from build123d import *

# Parameters (mm, degrees)
BOSS_EXTRUDE1_DEPTH = 12.7
SKETCH2_R           = 6.35
CUT_EXTRUDE5_DEPTH  = 12.7
FILLET1_R           = 2.54
FILLET2_R           = 2.54
SKETCH3_R           = 6.35
CUT_EXTRUDE6_DEPTH  = 12.7


with BuildPart() as part:
    # Sketch1 → Boss-Extrude1 (new body)
    with BuildSketch(Plane(origin=(0, 0, 0), x_dir=(1, 0, 0), z_dir=(0, 1, 0))):
        Polygon((0, 0), (203.2, 0), (101.6, 203.197957893), align=None)
    extrude(amount=BOSS_EXTRUDE1_DEPTH)

    # Sketch2 → Cut-Extrude5 (cut)
    with BuildSketch(Plane(origin=(0, 0, 0), x_dir=(1, 0, 0), z_dir=(0, 1, 0))):
        with Locations(Location((101.6, 165.097957893, 0), (0, 0, 270))):
            Circle(SKETCH2_R)
        Polygon((38.1, 25.4), (88.9, 25.4), (88.9, 127), align=None)
        Polygon((165.1, 25.4), (114.3, 25.4), (114.3, 127), align=None)
    extrude(amount=CUT_EXTRUDE5_DEPTH, mode=Mode.SUBTRACT)

    # Fillet1
    fillet1_edges = [part.edges().sort_by_distance(p)[0] for p in [
        (101.6, 6.35, -203.197957893),
        (203.2, 6.35, 0),
        (0, 6.35, 0),
    ]]
    fillet(fillet1_edges, radius=FILLET1_R)

    # Fillet2
    fillet2_edges = [part.edges().sort_by_distance(p)[0] for p in [
        (38.1, 6.35, -25.4),
        (88.9, 6.35, -25.4),
        (88.9, 6.35, -127),
        (165.1, 6.35, -25.4),
        (114.3, 6.35, -127),
        (114.3, 6.35, -25.4),
    ]]
    fillet(fillet2_edges, radius=FILLET2_R)

    # Sketch3 → Cut-Extrude6 (cut)
    with BuildSketch(Plane(origin=(0, 12.7, 0), x_dir=(1, 0, 0), z_dir=(0, 1, 0))):
        with Locations(Location((101.6, 88.9, 0), (0, 0, 270))):
            Circle(SKETCH3_R)
    extrude(amount=-CUT_EXTRUDE6_DEPTH, mode=Mode.SUBTRACT)


solid = part.part
Input: part model. Units: mm. Frame: model coordinates. A direction names the side the tool comes from. Give positions to 0.01 mm unless a question says otherwise; leave off trailing zeros. Order: outer loops, then holes, each group sorted by start corner. A loop starts at its lowest first (then second) coordinate and runs counter-clockwise, first axis right, second up. Notation, with made-up numbers: (-37, 28.5) -> (-15, 28.5) arc R35 cw to (-15, 65.5) -> close; hole circle Ø8 at (61, -14.75). An arc over 180 degrees is marked (long way). Use one line per item in the form item = value.
1) First-contact query: pin 1 Ø4 at (y, z) = (8, -60.5) entering from -X; pin 2 Ø1 at (y, z) = (10.5, -30) entering from -X; pin 3 Ø6 at (y, z) = (5.5, -165.5) entering from -X; pin 4 Ø11.5 at (x, z) = (101.6, -165.1) entering from +Y. Flat tips, straight axial feed; report the tip coordinate or a pass-through.
Response values:
pin_1 = 29.25
pin_2 = 14.75
pin_3 = 81.25
pin_4 = through
2) Mould query, pull axis X, two halves, no side actions, for faces 1 (the flat face through (100, 6, 0)), 2 (the flat face through (51.266, 6.261, -102.53)), 3 (the flat face through (153.3, 6.3, -99.8)), 4 (the flat face through (62.3, 6.3, -73.8)). Classes: pulls with the +X half, pulls with the -X half, needs draft (parallel to the pull), parting line crosses it, or undercut.
Response values:
face_1 = needs draft
face_2 = pulls with the -X half
face_3 = pulls with the +X half
face_4 = undercut
3) Section B-B, the plane y = 8. Return loops of the section in (x, z).
Response values:
outline = (1.84, -3.68) -> (99.33, -198.65) arc R2.54 ccw to (103.87, -198.65) -> (201.36, -3.68) arc R2.54 ccw to (199.09, 0) -> (4.11, 0) arc R2.54 ccw to start; hole (39.94, -29.08) -> (84.09, -117.38) arc R2.54 ccw to (88.9, -116.24) -> (88.9, -27.94) arc R2.54 ccw to (86.36, -25.4) -> (42.21, -25.4) arc R2.54 ccw to start; hole circle Ø12.7 at (101.6, -165.1); hole circle Ø12.7 at (101.6, -88.9); hole (114.3, -116.24) arc R2.54 ccw to (119.11, -117.38) -> (163.26, -29.08) arc R2.54 ccw to (160.99, -25.4) -> (116.84, -25.4) arc R2.54 ccw to (114.3, -27.94) -> close
4) Reachability of faces 5 (the flat face through (101, 0, -71)), 6 (the flat face through (140.9, 6.3, -73.8)) from +Z, -Z, +X, -X, +Y, -Y: full face, straight path, thin tool, end or side. Return the list, or none.
Response values:
face_5 = +Z, -Z, +X, -X, -Y
face_6 = +Y, -Y
5) Section C-C, the plane z = -47. Return loops of the section in (x, y).
Response values:
outline = (23.5, 0) -> (48.9, 0) -> (48.9, 12.7) -> (23.5, 12.7) -> close; (88.9, 0) -> (114.3, 0) -> (114.3, 12.7) -> (88.9, 12.7) -> close; (154.3, 0) -> (179.7, 0) -> (179.7, 12.7) -> (154.3, 12.7) -> close
6) Section D-D, the plane z = -88.9. Return loops of the section in (x, y).
Response values:
outline = (44.45, 0) -> (69.85, 0) -> (69.85, 12.7) -> (44.45, 12.7) -> close; (88.9, 0) -> (95.25, 0) -> (95.25, 12.7) -> (88.9, 12.7) -> close; (107.95, 0) -> (114.3, 0) -> (114.3, 12.7) -> (107.95, 12.7) -> close; (133.35, 0) -> (158.75, 0) -> (158.75, 12.7) -> (133.35, 12.7) -> close
7) Line query: probe 1 along X at (y, z) = (8.5, -90); probe 2 along X at (y, z) = (1.75, -27); probe 3 along X at (y, z) = (5.5, -71). Output: solid intervals per line, ascending.
Response values:
probe_1 = 45 to 70.4, 88.9 to 95.35, 107.85 to 114.3, 132.8 to 158.2
probe_2 = 13.5 to 39.85, 88.72 to 114.48, 163.35 to 189.7
probe_3 = 35.5 to 60.9, 88.9 to 114.3, 142.3 to 167.7
8) Section A-A, the plane x = 101.6. Return loops of the section in (y, z), and give its area (3 significant figures).
Response values:
outline = (0, -200.06) -> (12.7, -200.06) -> (12.7, -171.45) -> (0, -171.45) -> close; (0, -158.75) -> (12.7, -158.75) -> (12.7, -95.25) -> (0, -95.25) -> close; (0, -82.55) -> (12.7, -82.55) -> (12.7, 0) -> (0, 0) -> close
area = 2,220 mm^2
